Build history of the part. All positions in model axes, mm. Give positions to 0.01 mm unless a question says otherwise; leave off trailing zeros. Write each loop counter-clockwise with the first axis right and the second up, starting at its lowest first coordinate (ties: lowest second). Pieces come first, ordered by that corner, then holes. Notation, with made-up numbers: (3, 11.5) -> (38, 11.5) arc R16 ccw to (38, 36.5) -> close; hole circle Ø5 at (35.5, 44.5). An arc over 180 degrees is marked (long way). Put each result on its own line as item: value. Start each with the question number.
Item 1: Flat gauge pins, fed straight in: pin 1 Ø5.5 at (x, y) = (-15, 15) entering from +Z; pin 2 Ø12 at (y, z) = (37, -12) entering from +X; pin 3 Ø4 at (x, y) = (15.5, -15.5) entering from +Z; pin 4 Ø10 at (y, z) = (-43.5, 11.5) entering from +X. Where does each tip first touch, or does it go through?
Item 2: Slice it at A-A, the plane y = 15.5. List the corners of the cut face in (x, z).
Item 3: Drill centre lines: line 1 along Y through (x, z) = (-15.5, 13.75); line 2 along Y through (x, z) = (-15, 18); line 3 along X through (y, z) = (40, 9). Where is each one in solid material? Low to high.
Item 4: Slice it at C-C, the plane z = -18. List the corners of the cut face in (x, y), plus the area to 3 significant figures.
Item 5: Slice it at D-D, the plane x = -11.5. List the corners of the cut face in (y, z).
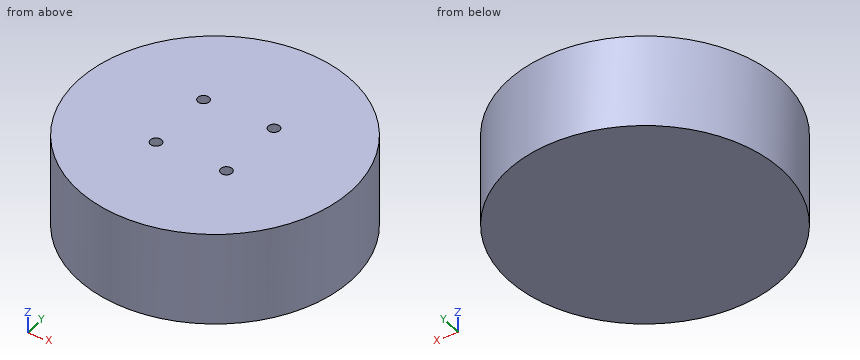
```python
from build123d import *

# Parameters (mm, degrees)
SKETCH1_R           = 60
BOSS_EXTRUDE1_DEPTH = 20.5
SKETCH2_R           = 2.5
CUT_EXTRUDE1_DEPTH  = 10


with BuildPart() as part:
    # Sketch1 → Boss-Extrude1 (new, symmetric)
    with BuildSketch(Plane.XY):
        Circle(SKETCH1_R)
    extrude(amount=BOSS_EXTRUDE1_DEPTH, both=True)

    # Sketch2 → Cut-Extrude1 (cut)
    with BuildSketch(Plane.XY.offset(20.5)):
        with Locations((-15.5, 15.5)):
            Circle(SKETCH2_R)
        with Locations((15.5, 15.5)):
            Circle(SKETCH2_R)
        with Locations((15.5, -15.5)):
            Circle(SKETCH2_R)
        with Locations((-15.5, -15.5)):
            Circle(SKETCH2_R)
    extrude(amount=-CUT_EXTRUDE1_DEPTH, mode=Mode.SUBTRACT)


solid = part.part
```
Values follow:
1. pin 1: z = 20.5
1. pin 2: x = 51.37
1. pin 3: z = 10.5
1. pin 4: x = 46.02
2. outline: (-57.96, -20.5) -> (57.96, -20.5) -> (57.96, 20.5) -> (18, 20.5) -> (18, 10.5) -> (13, 10.5) -> (13, 20.5) -> (-13, 20.5) -> (-13, 10.5) -> (-18, 10.5) -> (-18, 20.5) -> (-57.96, 20.5) -> close
3. line 1: -57.96 to -18, -13 to 13, 18 to 57.96
3. line 2: -58.09 to -17.95, -13.05 to 13.05, 17.95 to 58.09
3. line 3: -44.72 to 44.72
4. outline: circle Ø120 at (0, 0)
4. area: 11,300 mm2
5. outline: (-58.89, -20.5) -> (58.89, -20.5) -> (58.89, 20.5) -> (-58.89, 20.5) -> close
